CAD build for the part. Positions are in the model's coordinates, mm. Face numbers are marked on the shaded views. A direction names the side the tool comes from. Give positions to 0.01 mm unless a question says otherwise; leave off trailing zeros. Order: outer loops, then holes, each group sorted by start corner. A loop starts at its lowest first (then second) coordinate and runs counter-clockwise, first axis right, second up.
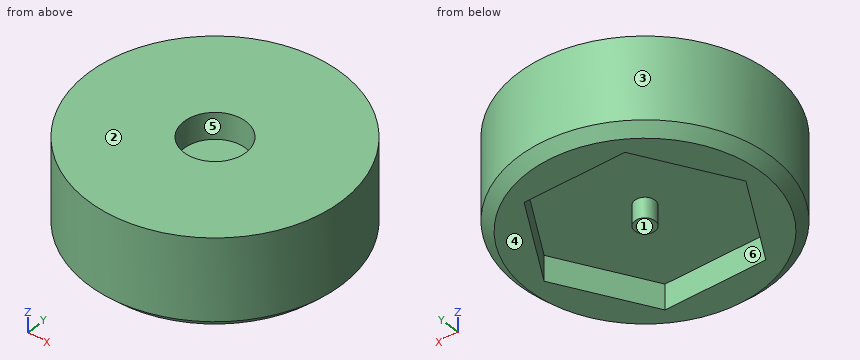
```python
from build123d import *

# Parameters (mm, degrees)
ESQUISSE1_R        = 12.5
BOSS_EXTRU_1_DEPTH = 2.5
ESQUISSE2_R        = 12.5
BOSS_EXTRU_2_DEPTH = 4
ESQUISSE3_R        = 1
BOSS_EXTRU_3_DEPTH = 2
CHANFREIN1_SIZE    = 1
ESQUISSE4_R        = 12.5
ESQUISSE4_R_2      = 3.05
BOSS_EXTRU_4_DEPTH = 2.6


with BuildPart() as part:
    # Esquisse1 → Boss.-Extru.1 (new body)
    with BuildSketch(Plane.XY):
        Circle(ESQUISSE1_R)
        Polygon((-4.936344802, -8.55), (4.936344802, -8.55), (9.872689603, 0), (4.936344802, 8.55), (-4.936344802, 8.55), (-9.872689603, 0), align=None, mode=Mode.SUBTRACT)
    extrude(amount=BOSS_EXTRU_1_DEPTH)

    # Esquisse2 → Boss.-Extru.2 (add)
    with BuildSketch(Plane.XY.offset(2.5)):
        Circle(ESQUISSE2_R)
    extrude(amount=BOSS_EXTRU_2_DEPTH)

    # Esquisse3 → Boss.-Extru.3 (add)
    with BuildSketch(Plane(origin=(0, 0, 2.5), x_dir=(-1, 0, 0), z_dir=(0, 0, -1))):
        with Locations(Location((0, 0, 0), (0, 0, 180))):
            Circle(ESQUISSE3_R)
    extrude(amount=BOSS_EXTRU_3_DEPTH)

    # Chanfrein1
    chanfrein1_edges = [part.edges().sort_by_distance(p)[0] for p in [
        (-12.5, 0, 0),
    ]]
    chamfer(chanfrein1_edges, length=CHANFREIN1_SIZE)

    # Esquisse4 → Boss.-Extru.4 (add)
    with BuildSketch(Plane.XY.offset(6.5)):
        Circle(ESQUISSE4_R)
        Circle(ESQUISSE4_R_2, mode=Mode.SUBTRACT)
    extrude(amount=BOSS_EXTRU_4_DEPTH)


solid = part.part
```
Item 1: Wall check: L1, parallel to Y at x = 0, z = 7.5; L2, parallel to Z at x = -3, y = 6.5; L3, parallel to X at y = -0.25, z = 3.25. Give the ranges that are in metal, low to high.
Item 2: Slice it at B-B (x = 0). Give the cut face in (y, z), and give its area (3 significant figures).
Item 3: Slice it at C-C (z = 8.25). Give the cut face in (x, y), and give its area (3 significant figures).
Item 4: Tool access for the marked faces 4, 5 and 6: list every direction of +Z, -Z, +X, -X, +Y, -Y with a clear straight run to the whole face (end or side of a thin tool).
Item 5: Slice it at A-A (z = 2). Give the cut face in (x, y), and give its area (3 significant figures).
Item 6: Drop flat-ended pins along their axis: pin 1 Ø5 at (x, z) = (-8, 5.5) entering from +Y (3 decimals); pin 2 Ø10 at (x, y) = (3.5, -6.5) entering from -Z; pin 3 Ø10 at (x, y) = (0, 0) entering from -Z; pin 4 Ø1.2 at (x, z) = (1.5, 0.5) entering from +Y. Give the stop position or say it passes through.
Item 7: Two-plate mould, pull along X, no slides. Class the marked faces 1, 2 and 3: released by +X, released by -X, zero draft, split by the parting line, or undercut.
A:
1. L1: y = -12.5 to -3.05, 3.05 to 12.5
1. L2: z = 2.5 to 9.1
1. L3: x = -12.5 to 12.5
2. outline: (-12.5, 1) - (-11.5, 0) - (-8.55, 0) - (-8.55, 2.5) - (-1, 2.5) - (-1, 0.5) - (1, 0.5) - (1, 2.5) - (8.55, 2.5) - (8.55, 0) - (11.5, 0) - (12.5, 1) - (12.5, 9.1) - (3.05, 9.1) - (3.05, 6.5) - (-3.05, 6.5) - (-3.05, 9.1) - (-12.5, 9.1) - close
2. area: 172 mm2
3. outline: circle Ø25 at (0, 0); hole circle Ø6.1 at (0, 0)
3. area: 462 mm2
4. face 4: -Z, +X, -X, +Y, -Y
4. face 5: +Z
4. face 6: -Z
5. outline: circle Ø25 at (0, 0); circle Ø2 at (0, 0); hole (-9.87, 0) - (-4.94, -8.55) - (4.94, -8.55) - (9.87, 0) - (4.94, 8.55) - (-4.94, 8.55) - close
5. area: 241 mm2
6. pin 1: stops at y = 11.225
6. pin 2: stops at z = 0
6. pin 3: stops at z = 0.5
6. pin 4: stops at y = 12.45
7. face 1: undercut
7. face 2: zero draft
7. face 3: split by the parting line
